from build123d import *

# Parameters (mm, degrees)
SKETCH2_R           = 8
SKETCH2_R_2         = 6
SKETCH2_W           = 7.6
SKETCH2_H           = 24.4
BOSS_EXTRUDE1_DEPTH = 3


with BuildPart() as part:
    # Sketch2 → Boss-Extrude1 (new body)
    with BuildSketch(Plane.XY):
        with BuildLine():
            Line((81.032103119, 50.181312), (81.032103119, 60.181312))
            Line((81.032103119, 60.181312), (78.032103119, 60.181312))
            ThreePointArc((78.032103119, 60.181312), (75.569321499, 69.649967364), (67.936161846, 75.770065518))
            Line((67.936161846, 75.770065518), (63.389132962, 73.023833254))
            Line((63.389132962, 73.023833254), (52.27464227, 79.356930255))
            Line((52.27464227, 79.356930255), (50.074247047, 75.495269488))
            Line((50.074247047, 75.495269488), (42.709956252, 79.691482274))
            Line((42.709956252, 79.691482274), (36.212476018, 75.495269488))
            Line((36.212476018, 75.495269488), (29.342622159, 77.861804263))
            ThreePointArc((29.342622159, 77.861804263), (14.166162437, 80.849682425), (-1.279201176, 80.017163065))
            ThreePointArc((-1.279201176, 80.017163065), (2.677054283, 70.700200378), (8.902417187, 62.718809041))
            ThreePointArc((8.902417187, 62.718809041), (5.05730693, 41.181312), (8.902417187, 19.643814959))
            ThreePointArc((8.902417187, 19.643814959), (2.677054283, 11.662423622), (-1.279201176, 2.345460935))
            ThreePointArc((-1.279201176, 2.345460935), (14.166162437, 1.512941575), (29.342622159, 4.500819737))
            Line((29.342622159, 4.500819737), (36.212476018, 6.867354512))
            Line((36.212476018, 6.867354512), (42.709956252, 2.671141726))
            Line((42.709956252, 2.671141726), (50.074247047, 6.867354512))
            Line((50.074247047, 6.867354512), (52.27464227, 3.005693745))
            Line((52.27464227, 3.005693745), (63.389132962, 9.338790746))
            Line((63.389132962, 9.338790746), (67.936161846, 6.592558482))
            ThreePointArc((67.936161846, 6.592558482), (75.569321499, 12.712656636), (78.032103119, 22.181312))
            Line((78.032103119, 22.181312), (81.032103119, 22.181312))
            Line((81.032103119, 22.181312), (81.032103119, 32.181312))
            Line((81.032103119, 32.181312), (78.032103119, 32.181312))
            Line((78.032103119, 32.181312), (78.032103119, 50.181312))
            Line((78.032103119, 50.181312), (81.032103119, 50.181312))
        make_face()
        with Locations((23.507028058, 53.931312)):
            Circle(SKETCH2_R, mode=Mode.SUBTRACT)
        with Locations((43.507028058, 41.181312)):
            Circle(SKETCH2_R_2, mode=Mode.SUBTRACT)
        with Locations((23.507028058, 28.431312)):
            Circle(SKETCH2_R, mode=Mode.SUBTRACT)
        with Locations((64.432028058, 41.181312)):
            Rectangle(SKETCH2_W, SKETCH2_H, mode=Mode.SUBTRACT)
        with BuildLine():
            ThreePointArc((21.611730632, 74.586477389), (14.814545044, 76.765459524), (7.678288301, 76.612049032))
            ThreePointArc((7.678288301, 76.612049032), (9.811410227, 72.018941841), (13.580912618, 68.636975763))
            ThreePointArc((13.580912618, 68.636975763), (17.183726984, 72.168659356), (21.611730632, 74.586477389))
        make_face(mode=Mode.SUBTRACT)
        with BuildLine():
            ThreePointArc((7.678288301, 5.750574968), (9.811410227, 10.343682159), (13.580912618, 13.725648237))
            ThreePointArc((13.580912618, 13.725648237), (17.183726984, 10.193964644), (21.611730632, 7.776146611))
            ThreePointArc((21.611730632, 7.776146611), (14.814545044, 5.597164476), (7.678288301, 5.750574968))
        make_face(mode=Mode.SUBTRACT)
    extrude(amount=BOSS_EXTRUDE1_DEPTH)


solid = part.part
Work out the finished part from the listing and answer in its coordinate system (mm). A direction names the side the tool comes from. Round coordinates to 2 decimals unless told otherwise and drop trailing zeros. Write each loop counter-clockwise with the first axis right and the second up, starting at its lowest first coordinate (ties: lowest second). Pieces come first, ordered by that corner, then holes. Notation, with made-up numbers: (37, -22.75) - (67, -22.75) arc R27 ccw to (67, 1.25) - close; hole circle Ø10 at (-6.5, 54.5). An arc over 180 degrees is marked (long way). Answer in a Markdown table with one row per item. Add a question column.
1. A cutting plane is placed at B-B, the plane x = 6.5. Determine the outline of the cut face in (y, z).
2. A cutting plane is placed at A-A, the plane y = 57. Determine the outline of the cut face in (x, z).
3. Given pin 1 (21 mm diameter, centred on x = 23.51, y = 28.43, fed in from +Z); pin 2 (1.5 mm diameter, centred on x = 79, z = 1, fed in from -Y); pin 3 (0.9 mm diameter, centred on x = 79, z = 1, fed in from +Y); pin 4 (0.9 mm diameter, centred on y = 44.5, z = 1.5, fed in from +X), each flat-ended and moving along its own axis, determine where each tip first touches the part or whether it passes through.
4. For faces 1 (the flat face through (46.444, 77.564, 1.479)), 2 (the flat face through (46.34, 4.74, 1.48)), 3 (the flat face through (80, 32.181, 1)), 4 (the cylindrical face through (2.605, 70.823, 1.479)), determine the directions among +Z, -Z, +X, -X, +Y, -Y from which every point of the face is accessible in a straight line to the end or side of a thin tool.
5. A cutting plane is placed at D-D, the plane z = 2.4. Count the separate pieces of the cut face and the enclosed holes in it, and give its area (3 significant figures).
6. Find the intervals of material crossed by line 1 along X through (y, z) = (43, 2.35); line 2 along X through (y, z) = (44.5, 1.8); line 3 along Y through (x, z) = (19, 1.5), in increasing order. Write a range as from..to.
7. The mould has two halves that part along Y. Classify faces 5 (the cylindrical face through (27.199, 46.834, 1.479)), 6 (the flat face through (81.032, 55, 1)), 7 (the flat face through (65.631, 7.985, 1.479)), 8 (the cylindrical face through (14.91, 76.75, 1.48)): +Y half, -Y half, draft (parallel to the pull), parting line (faces both ways), or undercut.
8. A cutting plane is placed at C-C, the plane y = 43. Determine the outline of the cut face in (x, z), and give its area (3 significant figures).
Worked out:
| question | item | result |
|---|---|---|
| 1 | outline | (1.44, 0) - (17.05, 0) - (17.05, 3) - (1.44, 3) - close; (27.86, 0) - (54.5, 0) - (54.5, 3) - (27.86, 3) - close; (65.31, 0) - (80.92, 0) - (80.92, 3) - (65.31, 3) - close |
| 2 | outline | (7.1, 0) - (16.12, 0) - (16.12, 3) - (7.1, 3) - close; (30.9, 0) - (81.03, 0) - (81.03, 3) - (30.9, 3) - close |
| 3 | pin 1 | z = 3 |
| 3 | pin 2 | y = 22.18 |
| 3 | pin 3 | y = 60.18 |
| 3 | pin 4 | x = 78.03 |
| 4 | face 1 | +Z, -Z, +Y |
| 4 | face 2 | +Z, -Z, -Y |
| 4 | face 3 | +Z, -Z, +X |
| 4 | face 4 | +Z, -Z, -X |
| 5 | separate pieces | 1 |
| 5 | enclosed holes | 6 |
| 5 | area | 4,510 mm^2 |
| 6 | line 1 | 5.08..37.79, 49.22..60.63, 68.23..78.03 |
| 6 | line 2 | 5.15..38.51, 48.51..60.63, 68.23..78.03 |
| 6 | line 3 | 2.04..6.64, 9.01..21.82, 35.04..47.32, 60.54..73.35, 75.72..80.32 |
| 7 | face 5 | undercut |
| 7 | face 6 | draft |
| 7 | face 7 | -Y half |
| 7 | face 8 | undercut |
| 8 | outline | (5.08, 0) - (37.79, 0) - (37.79, 3) - (5.08, 3) - close; (49.22, 0) - (60.63, 0) - (60.63, 3) - (49.22, 3) - close; (68.23, 0) - (78.03, 0) - (78.03, 3) - (68.23, 3) - close |
| 8 | area | 162 mm^2 |
